Build history of the part. All positions in model axes, mm. A direction names the side the tool comes from. Round coordinates to 2 decimals unless told otherwise and drop trailing zeros. Write each loop counter-clockwise with the first axis right and the second up, starting at its lowest first coordinate (ties: lowest second). Pieces come first, ordered by that corner, then holes. Notation, with made-up numbers: M -34.5,-21.75 L 15.5,-21.75 A12 cw 15.5,-0.75 Z; hole C 81.25,35 d3. An arc over 180 degrees is marked long. Write item = value, one per line.
from build123d import *

# Parameters (mm, degrees)
SKETCH1_R              = 2.38125
BOSS_EXTRUDE1_DEPTH    = 12.7
F_10_CLEARANCE_HOLE1_D = 5.1054
FILLET1_R              = 12.7


with BuildPart() as part:
    # Sketch1 → Boss-Extrude1 (new body)
    with BuildSketch(Plane(origin=(0, 0, 0), x_dir=(0, 0, -1), z_dir=(1, 0, 0))):
        Polygon((0, 0), (0, 101.6), (-25.4, 101.6), (-25.4, 50.8), (-152.4, 50.8), (-152.4, 0), align=None)
        with Locations((-84.1375, 25.4)):
            Circle(SKETCH1_R, mode=Mode.SUBTRACT)
        with Locations((-55.5625, 25.4)):
            Circle(SKETCH1_R, mode=Mode.SUBTRACT)
        with Locations((-26.9875, 25.4)):
            Circle(SKETCH1_R, mode=Mode.SUBTRACT)
    extrude(amount=BOSS_EXTRUDE1_DEPTH)

    # #10 Clearance Hole1 (through all)
    with Locations(Plane(origin=(12.7, 0, 0), x_dir=(0, 0, -1), z_dir=(1, 0, 0))):
        with Locations((-19.05, 95.25), (-6.35, 95.25), (-6.35, 82.55), (-19.05, 82.55)):
            Hole(F_10_CLEARANCE_HOLE1_D / 2)

    # Fillet1
    fillet1_edges = [part.edges().sort_by_distance(p)[0] for p in [
        (6.35, 50.8, 25.4),
    ]]
    fillet(fillet1_edges, radius=FILLET1_R)


solid = part.part
1. Band-saw the part on A-A (y = 82.55). List the corners of the cut face in (x, z), plus the area to 3 significant figures.
Responses:
outline = M 0,0 L 12.7,0 L 12.7,3.8 L 0,3.8 Z; M 0,8.9 L 12.7,8.9 L 12.7,16.5 L 0,16.5 Z; M 0,21.6 L 12.7,21.6 L 12.7,25.4 L 0,25.4 Z
area = 193 mm²
2. Mould opens along Y. For faces 1 (the face through (6, 0, 77)), 2 (the face through (6.261, 92.758, 18.497)), 3 (the face through (6, 101.6, 13)) say: pulls with the +Y half, pulls with the -Y half, needs draft (parallel to the pull), parting line crosses it, or undercut.
Responses:
face_1 = pulls with the -Y half
face_2 = undercut
face_3 = pulls with the +Y half
3. Band-saw the part on C-C (x = 2.25). List the corners of the cut face in (y, z), plus the area to 3 significant figures.
Responses:
outline = M 0,0 L 101.6,0 L 101.6,25.4 L 63.5,25.4 A12.7 cw 50.8,38.1 L 50.8,152.4 L 0,152.4 Z; hole C 25.4,26.99 d4.76; hole C 25.4,55.56 d4.76; hole C 25.4,84.14 d4.76; hole C 82.55,6.35 d5.11; hole C 82.55,19.05 d5.11; hole C 95.25,6.35 d5.11; hole C 95.25,19.05 d5.11
area = 8,930 mm²
4. Band-saw the part on D-D (z = 93). List the corners of the cut face in (x, y).
Responses:
outline = M 0,0 L 12.7,0 L 12.7,50.8 L 0,50.8 Z
5. Flat gauge pins, fed straight in: pin 1 (4 mm diameter, centred on x = 7.5, z = 78, fed in from +Y); pin 2 (3 mm diameter, centred on y = 82.55, z = 6.35, fed in from -X) (3 decimals). Where does each tip first touch, or does it go through?
Responses:
pin_1 = 50.8
pin_2 = through
6. Probe probe 1 along Y at (x, z) = (7.5, 19.05); probe 2 along Z at (x, y) = (1.25, 94); probe 3 along Z at (x, y) = (5.25, 81). List the from-to ranges inside material, lowest first.
Responses:
probe_1 = 0 to 80, 85.1 to 92.7, 97.8 to 101.6
probe_2 = 0 to 4.12, 8.58 to 16.82, 21.28 to 25.4
probe_3 = 0 to 4.32, 8.38 to 17.02, 21.08 to 25.4
7. Tool access for faces 4 (the face through (0, 29, 60)), 5 (the face through (6, 83, 25.4)): list every direction of +Z, -Z, +X, -X, +Y, -Y with a clear straight run to the whole face (end or side of a thin tool).
Responses:
face_4 = +Z, -Z, -X, +Y, -Y
face_5 = +Z, +X, -X, +Y
8. Band-saw the part on B-B (z = 6.35). List the corners of the cut face in (x, y), plus the area to 3 significant figures.
Responses:
outline = M 0,0 L 12.7,0 L 12.7,80 L 0,80 Z; M 0,85.1 L 12.7,85.1 L 12.7,92.7 L 0,92.7 Z; M 0,97.8 L 12.7,97.8 L 12.7,101.6 L 0,101.6 Z
area = 1,160 mm²
